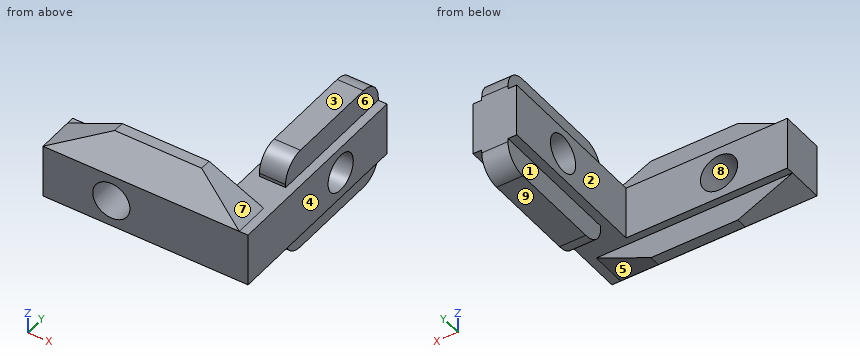
```python
from build123d import *
from OCP.BRepFilletAPI import BRepFilletAPI_MakeChamfer

# Parameters (mm, degrees)
EXTRUDE_1_DEPTH  = 4.9
EXTRUDE_2_DEPTH  = 35.9
CHAMFER_1_SIZE   = 10
CHAMFER_1_SIZE2  = 4.6
CHAMFER_2_SIZE   = 10
CHAMFER_2_SIZE_2 = 4.6
EXTRUDE_3_DEPTH  = 2.4


with BuildPart() as part:
    # 草图1 → 凸台-拉伸1 (new, symmetric)
    with BuildSketch(Plane.XY):
        Polygon((-37.5, 0), (0, 0), (0, 37.5), (-8, 37.5), (-8, 8), (-37.5, 8), align=None)
    extrude(amount=EXTRUDE_1_DEPTH, both=True)

    # 草图3 → 凸台-拉伸2 (add)
    with BuildSketch(Plane.ZY.offset(37.5)):
        Polygon((-4.9, 0), (-9.5, 4.6), (-9.5, 6.6), (-4.9, 6.6), align=None)
        Polygon((4.9, 6.6), (4.9, 0), (9.5, 4.6), (9.5, 6.6), align=None)
    extrude(amount=-EXTRUDE_2_DEPTH)

    # 倒角1: one chamfer whose edges measure the first distance from different faces: ONE call of the kernel's chamfer builder (chamfer() names one face for all edges)
    chamfer_1_edges_1 = [part.edges().sort_by_distance(p)[0] for p in [
        (-37.5, 5.6, 9.5),
    ]]
    chamfer_1_side_1 = [part.faces().sort_by_distance(p)[0] for p in [
        (-19.55, 5.6, 9.5),
    ]]
    chamfer_1_edges_2 = [part.edges().sort_by_distance(p)[0] for p in [
        (-37.5, 5.6, -9.5),
    ]]
    chamfer_1_side_2 = [part.faces().sort_by_distance(p)[0] for p in [
        (-19.55, 5.6, -9.5),
    ]]
    chamfer_1 = BRepFilletAPI_MakeChamfer(part.part.solid().wrapped)
    for e in chamfer_1_edges_1:
        chamfer_1.Add(CHAMFER_1_SIZE, CHAMFER_1_SIZE2, e.wrapped, chamfer_1_side_1[0].wrapped)  # the first distance lies on this face
    for e in chamfer_1_edges_2:
        chamfer_1.Add(CHAMFER_1_SIZE, CHAMFER_1_SIZE2, e.wrapped, chamfer_1_side_2[0].wrapped)  # the first distance lies on this face
    add(Compound.cast(chamfer_1.Shape()), mode=Mode.REPLACE)

    # 倒角2
    chamfer_2_edges_1 = [part.edges().sort_by_distance(p)[0] for p in [
        (-1.6, 5.6, 9.5),
    ]]
    chamfer_2_side_1 = [part.faces().sort_by_distance(p)[0] for p in [
        (-1.692, 5.6, 9.5),
    ]]
    chamfer_2_edges_2 = [part.edges().sort_by_distance(p)[0] for p in [
        (-1.6, 5.6, -9.5),
    ]]
    chamfer_2_side_2 = [part.faces().sort_by_distance(p)[0] for p in [
        (-1.692, 5.6, -9.5),
    ]]
    chamfer_2 = BRepFilletAPI_MakeChamfer(part.part.solid().wrapped)
    for e in chamfer_2_edges_1:
        chamfer_2.Add(CHAMFER_2_SIZE - 0.0001, CHAMFER_2_SIZE_2 - 0.0001, e.wrapped, chamfer_2_side_1[0].wrapped)
    for e in chamfer_2_edges_2:
        chamfer_2.Add(CHAMFER_2_SIZE - 0.0001, CHAMFER_2_SIZE_2 - 0.0001, e.wrapped, chamfer_2_side_2[0].wrapped)
    add(Compound.cast(chamfer_2.Shape()), mode=Mode.REPLACE)  # a hair under: the kernel refuses the full size

    # 草图5 → 凸台-拉伸3 (add, symmetric)
    with BuildSketch(Plane.ZY.offset(4)):
        with BuildLine():
            Line((-4.9, 37.5), (-5.5, 37.5))
            ThreePointArc((-5.5, 37.5), (-8.328427125, 36.328427125), (-9.5, 33.5))
            Line((-9.5, 33.5), (-9.5, 16.5))
            ThreePointArc((-9.5, 16.5), (-8.328427125, 13.671572875), (-5.5, 12.5))
            Line((-5.5, 12.5), (-4.9, 12.5))
            Line((-4.9, 12.5), (-4.9, 37.5))
        make_face()
        with BuildLine():
            Line((4.9, 12.5), (4.9, 37.5))
            Line((4.9, 37.5), (5.5, 37.5))
            ThreePointArc((5.5, 37.5), (8.328427125, 36.328427125), (9.5, 33.5))
            Line((9.5, 33.5), (9.5, 16.5))
            ThreePointArc((9.5, 16.5), (8.328427125, 13.671572875), (5.5, 12.5))
            Line((5.5, 12.5), (4.9, 12.5))
        make_face()
    extrude(amount=EXTRUDE_3_DEPTH, both=True)

    # 草图7 → M8 螺纹孔1 (revolve, cut)
    with BuildSketch(Plane(origin=(-25, 8, 0), x_dir=(0, 0, 1), z_dir=(1, 0, 0))):
        Polygon((0, 0), (0, 21.792926105), (3.4, 19.75), (3.4, 0), align=None)
    hole_wizard_m8_1 = revolve(axis=Axis((-25, 14.35, 0), (0, -1, 0)), mode=Mode.SUBTRACT)

    # 镜向1: M8 螺纹孔1 across plane
    add(hole_wizard_m8_1.mirror(Plane(origin=(0, 0, 0), x_dir=(0, 0, 1), z_dir=(-0.7071067811865477, -0.7071067811865475, 0))), mode=Mode.SUBTRACT)


solid = part.part
```
Check sheet for the modelled part. Datum: model origin and axes. Units: mm. Face numbers are marked on the shaded views. A direction names the side the tool comes from. Round coordinates to 2 decimals unless told otherwise and drop trailing zeros. Write each loop counter-clockwise with the first axis right and the second up, starting at its lowest first coordinate (ties: lowest second). Pieces come first, ordered by that corner, then holes. Notation, with made-up numbers: M 48,69 L 76,69 A12 ccw 76,79 Z; hole C -18,19.5 d5. An arc over 180 degrees is marked long. Write item = value, one per line. Start each with the question number.
1. Tool access check on the marked faces 1, 2, 3, 4 and 5. Record the directions out of +Z, -Z, +X, -X, +Y, -Y that give a thin tool (end or side, any length) a straight path to the whole face; none if there is none.
2. Release check for a two-part mould opening along Z. For the marked faces 6, 7, 8 and 9 record: pulls with the +Z half, pulls with the -Z half, needs draft (parallel to the pull), parting line crosses it, or undercut.
3. Section check A-A, the plane x = -25. Record the cut outline in (y, z).
4. Section check D-D, the plane y = 27. Record the cut outline in (x, z).
5. Section check B-B, the plane z = 0. Record the cut outline in (x, y), then the cut area to 3 significant figures.
6. Scan lines: line 1 (Z direction, x = -25, y = 6); line 2 (X direction, y = 3, z = 0); line 3 (Y direction, x = -4, z = 0). Record each from-to range of solid material in increasing order. Write a range as [from, to].
7. Gauge pin test, flat ends, axial feed: pin 1 (3.5 mm diameter, centred on y = 30, z = 7, fed in from +X); pin 2 (10 mm diameter, centred on y = 33.5, z = -2, fed in from -X); pin 3 (3.5 mm diameter, centred on x = -24, z = 6.5, fed in from +Y). Record the tip position at first contact, or that the pin passes through.
Results found:
q1.face_1 = -Z, -X, +Y
q1.face_2 = +Z, -Z, -X, +Y
q1.face_3 = +Z, +X, -X, +Y, -Y
q1.face_4 = +Z, -Z, +X, +Y, -Y
q1.face_5 = -Z, +X, -Y
q2.face_6 = needs draft
q2.face_7 = pulls with the +Z half
q2.face_8 = undercut
q2.face_9 = pulls with the -Z half
q3.outline = M 0,-4.9 L 4.6,-9.5 L 6.6,-9.5 L 6.6,-4.9 L 8,-4.9 L 8,-3.4 L 0,-3.4 Z; M 0,3.4 L 8,3.4 L 8,4.9 L 6.6,4.9 L 6.6,9.5 L 4.6,9.5 L 0,4.9 Z
q4.outline = M -8,-4.9 L -6.4,-4.9 L -6.4,-9.5 L -1.6,-9.5 L -1.6,-4.9 L 0,-4.9 L 0,-2.75 L -8,-2.75 Z; M -8,2.75 L 0,2.75 L 0,4.9 L -1.6,4.9 L -1.6,9.5 L -6.4,9.5 L -6.4,4.9 L -8,4.9 Z
q5.outline = M -37.5,0 L -28.4,0 L -28.4,8 L -37.5,8 Z; M -21.6,0 L 0,0 L 0,21.6 L -8,21.6 L -8,8 L -21.6,8 Z; M -8,28.4 L 0,28.4 L 0,37.5 L -8,37.5 Z
q5.area = 427 mm^2
q6.line_1 = [-9.5, -3.4], [3.4, 9.5]
q6.line_2 = [-37.5, -28.4], [-21.6, 0]
q6.line_3 = [0, 21.6], [28.4, 37.5]
q7.pin_1 = -1.6
q7.pin_2 = -8
q7.pin_3 = 8
